Autodesk Inventor part; units mm, degrees
ref_plane "YZ Plane" through (0, 0, 0) normal (1, 0, 0) x (0, 1, 0)
ref_plane "XZ Plane" through (0, 0, 0) normal (0, 1, 0) x (-1, 0, 0)
ref_plane "XY Plane" through (0, 0, 0) normal (0, 0, 1) x (1, 0, 0)
sketch "Sketch1" plane through (0, 0, 0) normal (0, 0, 1) x (1, 0, 0)
  line L0 (0, 0) -> (60, 0) construction
  line L1 (60, 0) -> (60, 60) construction
  line L2 (60, 60) -> (0, 60) construction
  line L3 (0, 3) -> (0, 0)
  line L4 (57, 60) -> (60, 60)
  line L5 (60, 60) -> (60, 30)
  line L6 (60, 0) -> (30, 0) construction
  line L7 (30, 0) -> (30, 30) construction
  line L8 (30, 30) -> (60, 30) construction
  line L9 (60, 30) -> (60, 0) construction
  arc A0 (30, 3) -> (57, 30) centre (30, 30) ccw
  line L10 (30, 3) -> (0, 3)
  line L11 (0, 0) -> (30, 0)
  line L12 (57, 30) -> (57, 60)
  line L13 (0, 60) -> (0, 30) construction
  line L14 (0, 3) -> (0, 0) construction
  arc A1 (30, 0) -> (60, 30) centre (30, 30) ccw
  arc A2 (30, 60) -> (0, 30) centre (30, 30) ccw
  dimension "d0" = 60
  dimension "d1" = 60
  dimension "d3" = 3
  dimension "d6" = 30
extrude "Extrusion2" add sketch "Sketch1" along normal blind 6
sketch "Sketch2" plane through (0, 0, 6) normal (0, 0, 1) x (1, 0, 0)
  line L0 (30, 3) -> (0, 3)
  line L1 (0, 0) -> (8, 0)
  line L2 (8, 0) -> (8, 3)
  line L3 (8, 3) -> (0, 3)
  line L4 (0, 3) -> (0, 0)
  dimension "d10" = 8
extrude "Extrusion3" add sketch "Sketch2" along normal blind 2
sketch "Sketch3" plane through (0, 3, 0) normal (0, 1, 0) x (1, 0, 0)
  circle A0 centre (4, -4) radius 2.15
  dimension "d13" = 4.3
extrude "Extrusion4" cut sketch "Sketch3" against normal through all
sketch "Sketch4" plane through (0, 0, 6) normal (0, 0, 1) x (1, 0, 0)
  line L0 (60, 30) -> (60, 60)
  line L1 (57, 60) -> (60, 60)
  line L2 (60, 60) -> (60, 52)
  line L3 (60, 52) -> (57, 52)
  line L4 (57, 52) -> (57, 60)
  point P0 (0, 0)
  dimension "d16" = 8
extrude "Extrusion5" add sketch "Sketch4" along normal blind 2
sketch "Sketch5" plane through (57, 30, 0) normal (-1, 0, 0) x (0, 0, 1)
  circle A0 centre (4, 26) radius 2.15
  point P0 (0, -30)
  dimension "d19" = 4.3
extrude "Extrusion6" cut sketch "Sketch5" against normal through all
sketch "Sketch6" plane through (0, 0, 0) normal (0, -1, 0) x (1, 0, 0)
  line L0 (30, 0) -> (0, 0)
  line L1 (8, 6) -> (30, 6)
  line L2 (8, 6) -> (8, 8)
  line L3 (0, 0) -> (0, 8)
  line L4 (9.5, 7.1237) -> (9.5, -0.5969) construction
  line L5 (9.5, 6) -> (12.5, 6)
  line L6 (12.5, 6) -> (12.5, 0)
  line L7 (12.5, 0) -> (9.5, 0)
  line L8 (9.5, 0) -> (9.5, 6)
  dimension "d23" = 1.5
  dimension "d24" = 3
extrude "Extrusion7" add sketch "Sketch6" along normal blind 4
sketch "Sketch7" plane through (60, 30, 0) normal (1, 0, 0) x (0, 0, -1)
  line L0 (0, 30) -> (0, 0)
  line L1 (-6, 22) -> (-8, 22)
  line L2 (-6, 0) -> (-6, 22)
  line L3 (-6, 20.5) -> (0, 20.5)
  line L4 (0, 20.5) -> (0, 17.5)
  line L5 (0, 17.5) -> (-6, 17.5)
  line L6 (-6, 17.5) -> (-6, 20.5)
  point P0 (0, -30)
  dimension "d27" = 3
  dimension "d28" = 1.5
extrude "Extrusion8" add sketch "Sketch7" along normal blind 4
fillet "Fillet1" radius 2 4 edges at (58.5, 52, 8) (58.5, 60, 8) (0, 1.5, 8) (8, 1.5, 8)
properties part number "BackNetHookLeft"
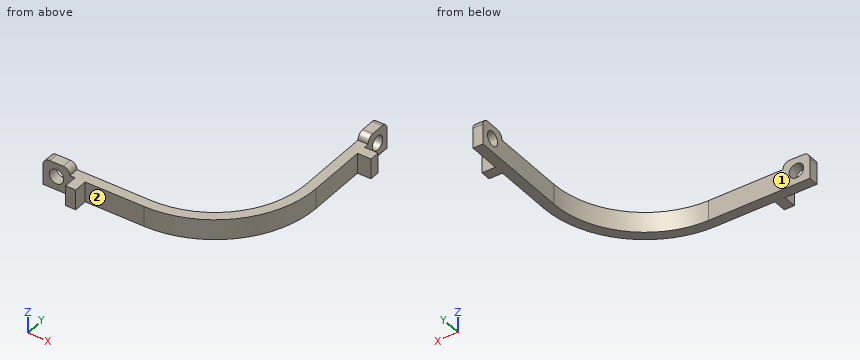
Could you check a few things on this model? Use its own coordinates, in mm. Face numbers are marked on the shaded views. A direction names the side the tool comes from. Coordinates: 2 decimals unless noted, no trailing zeros. Write each loop counter-clockwise with the first axis right and the second up, starting at its lowest first coordinate (ties: lowest second). Pieces come first, ordered by that corner, then holes. Notation, with made-up numbers: (76, 72) -> (117, 72) arc R22 cw to (117, 111) -> close; hole circle Ø11 at (2, -3.75). An arc over 180 degrees is marked (long way). One line per question, with ' | ' between items. Start each with the question number.
1. If we section it at D-D (y = 11): Please give me the cut outline in (x, z), and give its area (3 significant figures).
2. Please list where these lines run through material, in increasing order: line 1 along Z through (x, y) = (4, 2.4); line 2 along X through (y, z) = (44, 5.25); line 3 along X through (y, z) = (-0.5, 5.25).
3. For the marked faces 1 and 2, which set-ups out of +Z, -Z, +X, -X, +Y, -Y let a thin tool reach every point of the face, with its end or its side?
4. If we section it at A-A (x = 4): Please give me the cut outline in (y, z), and give its area (3 significant figures).
5. If we section it at B-B (z = 7): Please give me the cut outline in (x, y).
6. If we section it at C-C (z = 0.75): Please give me the cut outline in (x, y).
7. Will these pins go through, and if not, where does the flat tip stop? P1, Ø5, axis at x = 27.5, y = 5, coming from the +Z side; P2, Ø4.5, axis at y = -2, z = 3.5, coming from the -X side; P3, Ø17, axis at x = 26.5, y = 16, coming from the +Z side; P4, Ø2, axis at x = 63, z = 2.5, coming from the +Y side.
Return value:
1) outline: (49.18, 0) -> (53.22, 0) -> (53.22, 6) -> (49.18, 6) -> close | area: 24.2 mm²
2) line 1: z = 0 to 1.85, 6.15 to 8 | line 2: x = 57 to 60 | line 3: x = 9.5 to 12.5
3) face 1: +Z, -Z, -X, +Y | face 2: +Z, -Z, +X, -Y
4) outline: (0, 0) -> (3, 0) -> (3, 1.85) -> (0, 1.85) -> close; (0, 6.15) -> (3, 6.15) -> (3, 8) -> (0, 8) -> close | area: 11.1 mm²
5) outline: (0.27, 0) -> (7.73, 0) -> (7.73, 3) -> (0.27, 3) -> close; (57, 52.27) -> (60, 52.27) -> (60, 59.73) -> (57, 59.73) -> close
6) outline: (0, 0) -> (9.5, 0) -> (9.5, -4) -> (12.5, -4) -> (12.5, 0) -> (30, 0) arc R30 ccw to (60, 30) -> (60, 47.5) -> (64, 47.5) -> (64, 50.5) -> (60, 50.5) -> (60, 60) -> (57, 60) -> (57, 30) arc R27 cw to (30, 3) -> (0, 3) -> close
7) P1: stops at z = 6 | P2: stops at x = 0 | P3: passes through | P4: stops at y = 50.5
